Model file for the job. Use its own axes, mm. A direction names the side the tool comes from. Coordinates: 2 decimals unless noted, no trailing zeros. Order: outer loops, then holes, each group sorted by start corner. A loop starts at its lowest first (then second) coordinate and runs counter-clockwise, first axis right, second up.
from build123d import *

# Parameters (mm, degrees)
BODY_SKETCH_W                          = 230
BODY_SKETCH_H                          = 200
BODY_DEPTH                             = 4
MOUNTING_HOLES_OUTLINE_R               = 2.4
MOUNTING_HOLES_DEPTH                   = 4
SKETCH4_W                              = 230
SKETCH4_H                              = 18
CABLE_CUTOUTS_DEPTH                    = 1
SKETCH6_W                              = 28.5
SKETCH6_H                              = 104
DRIVER_EXTRUSION_DEPTH                 = 1
DRIVER_MOUNTING_HOLES_OUTLINE_R        = 2.25
DRIVER_MOUNTING_HOLES_DEPTH            = 5
DRIVER_PATTERN_COUNT                   = 4
DRIVER_PATTERN_PITCH                   = 53.5
SKETCH9_W                              = 5
SKETCH9_H                              = 3
CABLE_FIXIATOR_CUTOUT_DEPTH            = 153.449991801
CABLE_FIXIATOR_PATTERN_COUNT           = 5
CABLE_FIXIATOR_PATTERN_PITCH           = 51
CABLE_FIXIATOR_PATTERN_COPY_1_SKETCH_W = 5
CABLE_FIXIATOR_PATTERN_COPY_1_SKETCH_H = 3
CABLE_FIXIATOR_PATTERN_COPY_1_DEPTH    = 153.449991801
CABLE_FIXIATOR_PATTERN_COPY_2_SKETCH_W = 5
CABLE_FIXIATOR_PATTERN_COPY_2_SKETCH_H = 3
CABLE_FIXIATOR_PATTERN_COPY_2_DEPTH    = 153.449991801
CABLE_FIXIATOR_PATTERN_COPY_3_SKETCH_W = 5
CABLE_FIXIATOR_PATTERN_COPY_3_SKETCH_H = 3
CABLE_FIXIATOR_PATTERN_COPY_3_DEPTH    = 153.449991801
CABLE_FIXIATOR_PATTERN_COPY_4_SKETCH_W = 5
CABLE_FIXIATOR_PATTERN_COPY_4_SKETCH_H = 3
CABLE_FIXIATOR_PATTERN_COPY_4_DEPTH    = 153.449991801


# Read off the part's stored shape, not the designer's step: mounting_holes, driver_mounting_holes
with BuildPart() as part:
    # body_sketch → body (new body)
    with BuildSketch(Plane(origin=(0, 0, 0), x_dir=(1, 0, 0), z_dir=(0, 1, 0))):
        Rectangle(BODY_SKETCH_W, BODY_SKETCH_H)
    extrude(amount=BODY_DEPTH)

    # mounting_holes outline → mounting_holes (cut)
    with BuildSketch(Plane(origin=(0, 0, 0), x_dir=(1, 0, 0), z_dir=(0, 1, 0))):
        with Locations((110, -95)):
            Circle(MOUNTING_HOLES_OUTLINE_R)
        with Locations((-110, 95)):
            Circle(MOUNTING_HOLES_OUTLINE_R)
        with Locations((-110, -95)):
            Circle(MOUNTING_HOLES_OUTLINE_R)
        with Locations((110, 95)):
            Circle(MOUNTING_HOLES_OUTLINE_R)
    extrude(amount=MOUNTING_HOLES_DEPTH, mode=Mode.SUBTRACT)

    # Sketch4 → cable_cutouts (cut)
    with BuildSketch(Plane(origin=(0, 4, 0), x_dir=(1, 0, 0), z_dir=(0, 1, 0))):
        with Locations((0, 81)):
            Rectangle(SKETCH4_W, SKETCH4_H)
        with Locations((0, -41)):
            Rectangle(SKETCH4_W, SKETCH4_H)
    extrude(amount=-CABLE_CUTOUTS_DEPTH, mode=Mode.SUBTRACT)

    # Sketch6 → driver_extrusion (add)
    with BuildSketch(Plane(origin=(0, 4, 0), x_dir=(1, 0, 0), z_dir=(0, 1, 0))):
        with Locations((-80.75, 20)):
            Rectangle(SKETCH6_W, SKETCH6_H)
    driver_extrusion = extrude(amount=DRIVER_EXTRUSION_DEPTH)

    # driver_mounting_holes outline → driver_mounting_holes (cut)
    with BuildSketch(Plane(origin=(0, 0, 0), x_dir=(1, 0, 0), z_dir=(0, 1, 0))):
        with Locations((-85, -25)):
            Circle(DRIVER_MOUNTING_HOLES_OUTLINE_R)
        with Locations((-85, 65)):
            Circle(DRIVER_MOUNTING_HOLES_OUTLINE_R)
    driver_mounting_holes = extrude(amount=DRIVER_MOUNTING_HOLES_DEPTH, mode=Mode.SUBTRACT)

    # driver_pattern: driver_extrusion, driver_mounting_holes ×4
    with Locations(*[(i * DRIVER_PATTERN_PITCH, 0, 0) for i in range(1, DRIVER_PATTERN_COUNT)]):
        add(driver_extrusion)
        add(driver_mounting_holes, mode=Mode.SUBTRACT)

    # Sketch9 → cable_fixiator_cutout (cut, through all)
    with BuildSketch(Plane(origin=(0, 4, 0), x_dir=(1, 0, 0), z_dir=(0, 1, 0))):
        with Locations((-101.5, 93.5)):
            Rectangle(SKETCH9_W, SKETCH9_H)
        with Locations((-101.5, 68.5)):
            Rectangle(SKETCH9_W, SKETCH9_H)
    cable_fixiator_cutout = extrude(amount=-CABLE_FIXIATOR_CUTOUT_DEPTH, mode=Mode.SUBTRACT)

    # cable_fixiator_mirror: cable_fixiator_cutout across plane
    add(cable_fixiator_cutout.mirror(Plane.XY.offset(-20)), mode=Mode.SUBTRACT)

    # cable_fixiator_pattern: cable_fixiator_cutout ×5
    with Locations(*[(i * CABLE_FIXIATOR_PATTERN_PITCH, 0, 0) for i in range(1, CABLE_FIXIATOR_PATTERN_COUNT)]):
        add(cable_fixiator_cutout, mode=Mode.SUBTRACT)

    # cable_fixiator_pattern copy 1 sketch → cable_fixiator_pattern copy 1 (cut, through all)
    with BuildSketch(Plane(origin=(51, 4, -40), x_dir=(1, 0, 0), z_dir=(0, 1, 0))):
        with Locations((-101.5, -93.5)):
            Rectangle(CABLE_FIXIATOR_PATTERN_COPY_1_SKETCH_W, CABLE_FIXIATOR_PATTERN_COPY_1_SKETCH_H)
        with Locations((-101.5, -68.5)):
            Rectangle(CABLE_FIXIATOR_PATTERN_COPY_1_SKETCH_W, CABLE_FIXIATOR_PATTERN_COPY_1_SKETCH_H)
    extrude(amount=-CABLE_FIXIATOR_PATTERN_COPY_1_DEPTH, mode=Mode.SUBTRACT)

    # cable_fixiator_pattern copy 2 sketch → cable_fixiator_pattern copy 2 (cut, through all)
    with BuildSketch(Plane(origin=(102, 4, -40), x_dir=(1, 0, 0), z_dir=(0, 1, 0))):
        with Locations((-101.5, -93.5)):
            Rectangle(CABLE_FIXIATOR_PATTERN_COPY_2_SKETCH_W, CABLE_FIXIATOR_PATTERN_COPY_2_SKETCH_H)
        with Locations((-101.5, -68.5)):
            Rectangle(CABLE_FIXIATOR_PATTERN_COPY_2_SKETCH_W, CABLE_FIXIATOR_PATTERN_COPY_2_SKETCH_H)
    extrude(amount=-CABLE_FIXIATOR_PATTERN_COPY_2_DEPTH, mode=Mode.SUBTRACT)

    # cable_fixiator_pattern copy 3 sketch → cable_fixiator_pattern copy 3 (cut, through all)
    with BuildSketch(Plane(origin=(153, 4, -40), x_dir=(1, 0, 0), z_dir=(0, 1, 0))):
        with Locations((-101.5, -93.5)):
            Rectangle(CABLE_FIXIATOR_PATTERN_COPY_3_SKETCH_W, CABLE_FIXIATOR_PATTERN_COPY_3_SKETCH_H)
        with Locations((-101.5, -68.5)):
            Rectangle(CABLE_FIXIATOR_PATTERN_COPY_3_SKETCH_W, CABLE_FIXIATOR_PATTERN_COPY_3_SKETCH_H)
    extrude(amount=-CABLE_FIXIATOR_PATTERN_COPY_3_DEPTH, mode=Mode.SUBTRACT)

    # cable_fixiator_pattern copy 4 sketch → cable_fixiator_pattern copy 4 (cut, through all)
    with BuildSketch(Plane(origin=(204, 4, -40), x_dir=(1, 0, 0), z_dir=(0, 1, 0))):
        with Locations((-101.5, -93.5)):
            Rectangle(CABLE_FIXIATOR_PATTERN_COPY_4_SKETCH_W, CABLE_FIXIATOR_PATTERN_COPY_4_SKETCH_H)
        with Locations((-101.5, -68.5)):
            Rectangle(CABLE_FIXIATOR_PATTERN_COPY_4_SKETCH_W, CABLE_FIXIATOR_PATTERN_COPY_4_SKETCH_H)
    extrude(amount=-CABLE_FIXIATOR_PATTERN_COPY_4_DEPTH, mode=Mode.SUBTRACT)


solid = part.part
Q1. Cut at C-C, the plane z = 77. List the corners of the cut face in (x, y).
Established:
outline: (-115, 0) - (115, 0) - (115, 4) - (-115, 4) - close
Q2. Drop a flat-ended pin along its axis: P1, Ø4, axis at x = -78.5, z = 57.5, coming from the +Y side. Give the stop position or say it passes through.
Established:
P1: stops at y = 4
Q3. Mould opens along X. For faces 1 (the face through (-2, 3, -81)), 2 (the face through (-1, 4, -21)) say: pulls with the +X half, pulls with the -X half, needs draft (parallel to the pull), parting line crosses it, or undercut.
Established:
face 1: needs draft
face 2: undercut
Q4. Probe line 1 (X direction, y = 0.9, z = 95); line 2 (Z direction, x = -31.5, y = 3.1); line 3 (X direction, y = 2.35, z = 25). List the from-to ranges inside material, lowest first.
Established:
line 1: x = -115 to -112.4, -107.6 to 107.6, 112.4 to 115
line 2: z = -100 to -90, -72 to -67.25, -62.75 to 22.75, 27.25 to 32, 50 to 100
line 3: x = -115 to -87.25, -82.75 to -33.75, -29.25 to 19.75, 24.25 to 73.25, 77.75 to 115
Q5. Cut at B-B, the plane x = 85. List the corners of the cut face in (y, z), plus the area to 3 significant figures.
Established:
outline: (0, -100) - (4, -100) - (4, -90) - (3, -90) - (3, -72) - (5, -72) - (5, 32) - (3, 32) - (3, 50) - (4, 50) - (4, 100) - (0, 100) - close
area: 868 mm2
Q6. Cut at D-D, the plane z = 38. List the corners of the cut face in (x, y), plus the area to 3 significant figures.
Established:
outline: (-115, 0) - (115, 0) - (115, 3) - (-115, 3) - close
area: 690 mm2
Q7. Which spindle directions (+Z, -Z, +X, -X, +Y, -Y) get a long thin tool onto all of the face, cutting with end or side? Do faces 3 (the face through (-2, 3, 41)), 4 (the face through (-105, 4, -21)), 5 (the face through (-54, 4, -21)). Say none if no direction does.
Established:
face 3: +X, -X, +Y
face 4: +Z, -Z, -X, +Y
face 5: +Z, -Z, +Y
Q8. Cut at A-A, the plane z = -50. List the corners of the cut face in (x, y).
Established:
outline: (-115, 0) - (115, 0) - (115, 4) - (94, 4) - (94, 5) - (65.5, 5) - (65.5, 4) - (40.5, 4) - (40.5, 5) - (12, 5) - (12, 4) - (-13, 4) - (-13, 5) - (-41.5, 5) - (-41.5, 4) - (-66.5, 4) - (-66.5, 5) - (-95, 5) - (-95, 4) - (-115, 4) - close
